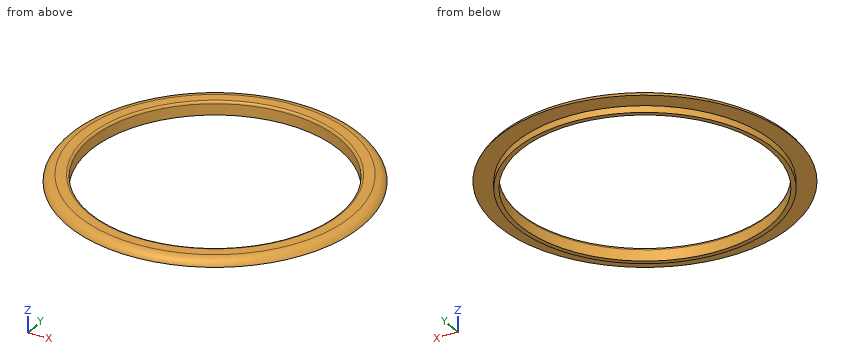
from build123d import *

# Parameters (mm, degrees)
F0_R     = 58
F0_R_2   = 56
F1_DEPTH = 3
F2_R     = 66
F2_R_2   = 58
F2_R_3   = 56
F3_DEPTH = 3
F5_R     = 1


# Not quite as in the source:
# - a fillet or chamfer that OpenCascade refuses, or shapes differently, is made with other operations: its cross-section is extruded or revolved along the edge and cut away or added


with BuildPart() as f1:
    # F0 (on Top) → F1 (new body)
    with BuildSketch(Plane.XY):
        Circle(F0_R)
        Circle(F0_R_2, mode=Mode.SUBTRACT)
    extrude(amount=F1_DEPTH)

    # F2 (on face) → F3 (join)
    with BuildSketch(Plane.XY.offset(3)):
        Circle(F2_R)
        Circle(F2_R_2, mode=Mode.SUBTRACT)
        Circle(F2_R_2)
        Circle(F2_R_3, mode=Mode.SUBTRACT)
    extrude(amount=F3_DEPTH)

    # F4: fillet of radius 5 on 1 edges, made by hand

    # F4_s1 → F4_t2 (revolve, cut)
    with BuildSketch(Plane.XZ):
        with BuildLine():
            ThreePointArc((66, 3), (64.1560370926, 5.1833001327), (61.417424305, 6))
            Line((61.417424305, 6), (66, 6))
            Line((66, 6), (66, 3))
        make_face()
    revolve(axis=Axis((0, 0, 6), (0, 0, 1)), mode=Mode.SUBTRACT)

    # F5
    f5_edges = [f1.edges().sort_by_distance(p)[0] for p in [
        (-56, 0, 6),
    ]]
    fillet(f5_edges, radius=F5_R)


solid = f1.part
The model under review builds one solid part; all positions refer to its coordinate system, in mm. Coordinates: 2 decimals unless noted, no trailing zeros. Loops run counter-clockwise (first coordinate to the right, second up) from the corner with the lowest first, then second, coordinate; pieces in that order, holes last. Notation, with made-up numbers: M 62.5,48 L 99.5,48 A24 ccw 99.5,74 Z; hole C 83,50 d4. An arc over 180 degrees is marked long. Put each result on its own line as item: value. Start each with the question number.
Q1. Add section C-C (z = 1.75). Write out the cut boundary in (x, y).
Q2. Add section A-A (y = 0). Write out the cut boundary in (x, z).
Q3. Clearance check with flat-ended pins moving along their axes: pin 1 (1 mm diameter, centred on x = -33, z = 5, fed in from +Y); pin 2 (2 mm diameter, centred on y = 25.5, z = 2.5, fed in from +X); pin 3 (1.5 mm diameter, centred on x = -43, y = 36, fed in from +Z). State where each tip first meets the part, or that it passes through.
Q4. Wall thickness on line 1 (Y direction, x = 0, z = 1.8); line 2 (Y direction, x = -36, z = 2); line 3 (X direction, y = -32, z = 0.5): over which ranges is each line inside the solid? List them lowest first.
Answers:
1. outline: C 0,0 d116; hole C 0,0 d112
2. outline: M -66,3 L -58,3 L -58,0 L -56,0 L -56,5 A1 ccw -57,6 L -61.42,6 A5 ccw Z; M 56,0 L 58,0 L 58,3 L 66,3 A5 ccw 61.42,6 L 57,6 A1 ccw 56,5 Z
3. pin 1: stops at y = 56.06
3. pin 2: stops at x = 61.23
3. pin 3: stops at z = 5.99
4. line 1: y = -58 to -56, 56 to 58
4. line 2: y = -45.48 to -42.9, 42.9 to 45.48
4. line 3: x = -48.37 to -45.96, 45.96 to 48.37
